Input: part model. Units: mm. Frame: model coordinates. Face numbers are marked on the shaded views. A direction names the side the tool comes from. Coordinates: 2 decimals unless noted, no trailing zeros. Order: outer loops, then holes, each group sorted by start corner. A loop starts at its lowest first (then second) coordinate and runs counter-clockwise, first axis right, second up. Notation, with made-up numbers: (45.5, -1) - (61.5, -1) arc R13 ccw to (61.5, 13) - close; hole circle Ø11 at (64.25, 32.5). An arc over 180 degrees is marked (long way). One line per question, with ' | ' between items. Start each with the question number.
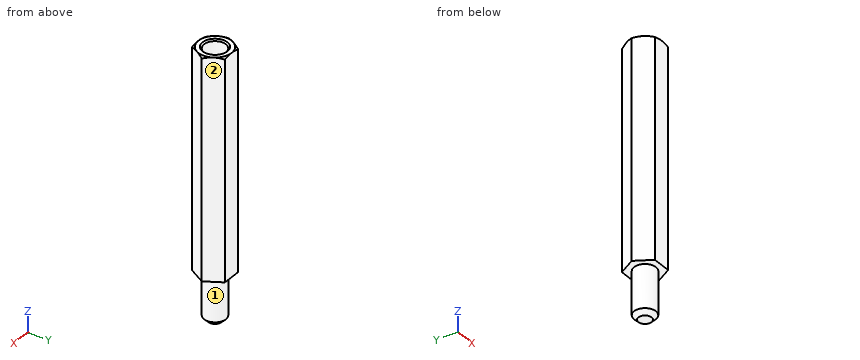
```python
from build123d import *

# Parameters (mm, degrees)
BOSS_EXTRUDE1_DEPTH     = 30
SKETCH2_R               = 1.5
CUT_EXTRUDE1_DEPTH      = 1
CUT_EXTRUDE1_DEPTH_BACK = 12
CHAMFER1_SIZE           = 0.2
SKETCH4_R               = 1.5
BOSS_EXTRUDE2_DEPTH     = 6.5
CHAMFER2_SIZE           = 0.6


with BuildPart() as part:
    # Sketch1 → Boss-Extrude1 (new body)
    with BuildSketch(Plane.XY):
        Polygon((2.621170222, 0), (1.310585111, 2.27), (-1.310585111, 2.27), (-2.621170222, 0), (-1.310585111, -2.27), (1.310585111, -2.27), align=None)
    extrude(amount=BOSS_EXTRUDE1_DEPTH)

    # Sketch2 → Cut-Extrude1 (cut, two sides)
    with BuildSketch(Plane.XY.offset(30)) as cut_extrude1_sk:
        Circle(SKETCH2_R)
    extrude(amount=CUT_EXTRUDE1_DEPTH, mode=Mode.SUBTRACT)
    extrude(cut_extrude1_sk.sketch, amount=-CUT_EXTRUDE1_DEPTH_BACK, mode=Mode.SUBTRACT)

    # Sketch3 → Cut-Revolve1 (revolve, cut)
    with BuildSketch(Plane(origin=(0, 0, 0), x_dir=(1, 0, 0), z_dir=(0, 1, 0))):
        Polygon((-2.621170222, -30), (-2.271170222, -30), (-2.621170222, -29.8), align=None)
    revolve(axis=Axis((0, 0, 18), (0, 0, 1)), mode=Mode.SUBTRACT)

    # Chamfer1
    chamfer1_edges = [part.edges().sort_by_distance(p)[0] for p in [
        (-1.5, 0, 30),
    ]]
    chamfer(chamfer1_edges, length=CHAMFER1_SIZE)

    # Sketch4 → Boss-Extrude2 (add)
    with BuildSketch(Plane(origin=(0, 0, 0), x_dir=(-1, 0, 0), z_dir=(0, 0, -1))):
        Circle(SKETCH4_R)
    extrude(amount=BOSS_EXTRUDE2_DEPTH)

    # Chamfer2
    chamfer2_edges = [part.edges().sort_by_distance(p)[0] for p in [
        (1.5, 0, -6.5),
    ]]
    chamfer(chamfer2_edges, length=CHAMFER2_SIZE)


solid = part.part
```
(1) Section A-A (z = 17). Output: boundary loops of the cut face in (x, y), then the cut area to 3 significant figures.
(2) Material intervals for line 1 along Y through (x, z) = (0, 21.25); line 2 along Z through (x, y) = (1.1, -1.4); line 3 along Y through (x, z) = (1.35, 23), sorted ascending. Write a range as from..to.
(3) Pin query (flat end, axial travel): pin 1 (1.5 mm diameter, centred on x = 0.5, y = 1, fed in from +Z). Return the tip coordinate at first contact, or that it passes through.
(4) Reachability of the marked faces 1 and 2 from +Z, -Z, +X, -X, +Y, -Y: full face, straight path, thin tool, end or side. Return the list, or none.
Worked answers:
1) outline: (-2.62, 0) - (-1.31, -2.27) - (1.31, -2.27) - (2.62, 0) - (1.31, 2.27) - (-1.31, 2.27) - close | area: 17.9 mm²
2) line 1: y = -2.27..-1.5, 1.5..2.27 | line 2: z = 0..30 | line 3: y = -2.2..-0.65, 0.65..2.2
3) pin 1: stops at z = 30
4) face 1: -Z | face 2: +Z, -Z, +X, +Y
